Read the model definition and answer for the solid it produces. Units are mm, in the model's axes. A direction names the side the tool comes from. Coordinates: 2 decimals unless noted, no trailing zeros. Write item = value, one per line.
from build123d import *

# Parameters (mm, degrees)
SKETCH_1_W          = 158
SKETCH_1_H          = 200
EXTRUDE_1_DEPTH     = 10
SKETCH_2_RX         = 12.510915337
SKETCH_2_RY         = 9.050449393
SKETCH_2_RX_2       = 5.182590636
SKETCH_2_RY_2       = 3.452265776
SKETCH_2_RX_3       = 5.641827611
SKETCH_2_RX_4       = 5.141705424
SKETCH_2_RX_5       = 4.748897539
CUT_EXTRUDE_1_DEPTH = 2


with BuildPart() as part:
    # 草圖1 → 填料-伸長1 (new body)
    with BuildSketch(Plane.XY):
        with Locations((79, 100)):
            Rectangle(SKETCH_1_W, SKETCH_1_H)
    extrude(amount=EXTRUDE_1_DEPTH)

    # 草圖2 → 除料-伸長1 (cut)
    with BuildSketch(Plane.XY.offset(10)):
        with Locations((73.143826864, 161.889102465)):
            Ellipse(SKETCH_2_RX, SKETCH_2_RY)
        with Locations(Location((55.175550619, 169.508366321), (0, 0, -29.658527045))):
            Ellipse(SKETCH_2_RX_2, SKETCH_2_RY_2)
        with Locations(Location((64.548995649, 177.167911946), (0, 0, -57.180664348))):
            Ellipse(SKETCH_2_RX_3, SKETCH_2_RY_2)
        with Locations(Location((75.880101936, 177.650055904), (0, 0, 90))):
            Ellipse(SKETCH_2_RX_4, SKETCH_2_RY_2)
        with Locations(Location((88.871515974, 172.008159222), (0, 0, -128.304052106))):
            Ellipse(SKETCH_2_RX_5, SKETCH_2_RY_2)
    extrude(amount=-CUT_EXTRUDE_1_DEPTH, mode=Mode.SUBTRACT)


solid = part.part
1) For faces 1 (the face through (65, 177, 8)), 2 (the face through (158, 99, 5)), determine the directions among +Z, -Z, +X, -X, +Y, -Y from which every point of the face is accessible in a straight line to the end or side of a thin tool.
Returned:
face_1 = +Z
face_2 = +Z, -Z, +X, +Y, -Y
2) Determine the mould class of faces 3 (the face through (0, 99, 5)), 4 (the face through (73, 162, 8)), 5 (the face through (78, 0, 5)) for opening direction Y: pulls with the +Y half, pulls with the -Y half, needs draft (parallel to the pull), parting line crosses it, or undercut.
Returned:
face_3 = needs draft
face_4 = undercut
face_5 = pulls with the -Y half
3) A flat-ended cylindrical pin translates along its axis: pin 1 Ø9 at (x, y) = (76, 164.5) entering from +Z. Find the tip coordinate at first contact, or state that the pin passes through.
Returned:
pin_1 = 8
4) A straight line is drawn through the part: line 1 along Y through (x, z) = (90, 9). Find the intervals that lie inside material, in ascending order. Write a range as from..to.
Returned:
line_1 = 0..168.44, 176.3..200
